```python
from build123d import *

# Parameters (mm, degrees)
F0_W          = 15
F0_H          = 15
F0_W_2        = 11
F0_H_2        = 11
F1_DEPTH      = 7.5
F1_DEPTH_BACK = 7.5
F2_W          = 11
F2_H          = 11
F3_DEPTH      = 25
F4_W          = 11
F4_H          = 11
F5_DEPTH      = 15.001


# Not quite as in the source:
# - the program builds the solid bodies; features that only make, move or delete a surface that nothing else refers to are left out


with BuildPart() as f1:
    # F0 (on Top) → F1 (new body, two sides)
    with BuildSketch(Plane.XY) as f1_sk:
        Rectangle(F0_W, F0_H)
        Rectangle(F0_W_2, F0_H_2, mode=Mode.SUBTRACT)
    extrude(amount=F1_DEPTH)
    extrude(f1_sk.sketch, amount=-F1_DEPTH_BACK)

    # F2 (on face) → F3 (cut)
    with BuildSketch(Plane.XZ.offset(7.5)):
        Rectangle(F2_W, F2_H)
    extrude(amount=-F3_DEPTH, mode=Mode.SUBTRACT)

    # F4 (on face) → F5 (cut, through all)
    with BuildSketch(Plane.YZ.offset(7.5)):
        Rectangle(F4_W, F4_H)
    extrude(amount=-F5_DEPTH, mode=Mode.SUBTRACT)


solid = f1.part
```
For this review, take the finished solid that the model builds, in its own axes (mm). A direction names the side the tool comes from. Round coordinates to 2 decimals unless told otherwise and drop trailing zeros. Loops run counter-clockwise (first coordinate to the right, second up) from the corner with the lowest first, then second, coordinate; pieces in that order, holes last.
Q1. To check wall thickness, follow line 1 along Z through (x, y) = (-2.25, 6). State the ranges of the line that lie inside material, in increasing order.
Result sheet:
line 1: z = -7.5 to -5.5, 5.5 to 7.5
Q2. Add section C-C on x = -6.5. Write out the cut boundary in (y, z).
Result sheet:
outline: (-7.5, -7.5) - (7.5, -7.5) - (7.5, 7.5) - (-7.5, 7.5) - close; hole (-5.5, -5.5) - (5.5, -5.5) - (5.5, 5.5) - (-5.5, 5.5) - close
Q3. Machinability: for faces 4 (the face through (7, 5.5, 0)), 5 (the face through (7.5, -7, 0)), 6 (the face through (0, 6, -5.5)), 7 (the face through (0, 5.5, -6)), which of the approach directions +Z, -Z, +X, -X, +Y, -Y give a long, thin tool a straight path to every point of the face, cutting with its end or side? Answer none if there is none.
Result sheet:
face 4: +X, -X
face 5: +Z, -Z, +X, +Y, -Y
face 6: +Y, -Y
face 7: +Z, -Z
Q4. Add section A-A on z = 2.25. Write out the cut boundary in (x, y), plus the area to 3 significant figures.
Result sheet:
outline: (-7.5, -7.5) - (-5.5, -7.5) - (-5.5, -5.5) - (-7.5, -5.5) - close; (-7.5, 5.5) - (-5.5, 5.5) - (-5.5, 7.5) - (-7.5, 7.5) - close; (5.5, -7.5) - (7.5, -7.5) - (7.5, -5.5) - (5.5, -5.5) - close; (5.5, 5.5) - (7.5, 5.5) - (7.5, 7.5) - (5.5, 7.5) - close
area: 16.0 mm2
Q5. Mouldability with a two-part tool opening along Z and no side actions: class faces 1 (the face through (-7, 0, 7.5)), 2 (the face through (7, 0, -5.5)), 3 (the face through (-7, 7.5, 0)) as +Z half, -Z half, draft (parallel to the pull), parting line (faces both ways), or undercut.
Result sheet:
face 1: +Z half
face 2: undercut
face 3: draft
